CAD build for the part. Positions are in the model's coordinates, mm. A direction names the side the tool comes from. Round coordinates to 2 decimals unless told otherwise and drop trailing zeros. Loops run counter-clockwise (first coordinate to the right, second up) from the corner with the lowest first, then second, coordinate; pieces in that order, holes last.
from build123d import *

# Parameters (mm, degrees)
SKETCH2_W           = 6.35
SKETCH2_H           = 152.4
SKETCH2_H_2         = 6.35
SKETCH2_W_2         = 25.4
SKETCH2_W_3         = 3.175
BOSS_EXTRUDE1_DEPTH = 152.4
SKETCH3_W           = 228.6
SKETCH3_H           = 165.1
BOSS_EXTRUDE2_DEPTH = 12.7


with BuildPart() as part:
    # Sketch2 → Boss-Extrude1 (new body)
    with BuildSketch(Plane.XY):
        with Locations((-111.125, 79.375)):
            Rectangle(SKETCH2_W, SKETCH2_H)
        with Locations((-111.125, 158.75)):
            Rectangle(SKETCH2_W, SKETCH2_H_2)
        with Locations((-95.25, 158.75)):
            Rectangle(SKETCH2_W_2, SKETCH2_H_2)
        with Locations((-80.9625, 158.75)):
            Rectangle(SKETCH2_W_3, SKETCH2_H_2)
        with Locations((-76.2, 158.75)):
            Rectangle(SKETCH2_W, SKETCH2_H_2)
        with Locations((-71.4375, 158.75)):
            Rectangle(SKETCH2_W_3, SKETCH2_H_2)
        with Locations((-57.15, 158.75)):
            Rectangle(SKETCH2_W_2, SKETCH2_H_2)
        with Locations((-42.8625, 158.75)):
            Rectangle(SKETCH2_W_3, SKETCH2_H_2)
        with Locations((-42.8625, 152.4)):
            Rectangle(SKETCH2_W_3, SKETCH2_H_2)
        with Locations((-38.1, 158.75)):
            Rectangle(SKETCH2_W, SKETCH2_H_2)
        with Locations((-33.3375, 158.75)):
            Rectangle(SKETCH2_W_3, SKETCH2_H_2)
        with Locations((-33.3375, 152.4)):
            Rectangle(SKETCH2_W_3, SKETCH2_H_2)
        with Locations((-19.05, 158.75)):
            Rectangle(SKETCH2_W_2, SKETCH2_H_2)
        with Locations((-4.7625, 158.75)):
            Rectangle(SKETCH2_W_3, SKETCH2_H_2)
        with Locations((-4.7625, 152.4)):
            Rectangle(SKETCH2_W_3, SKETCH2_H_2)
        with Locations((0, 158.75)):
            Rectangle(SKETCH2_W, SKETCH2_H_2)
        with Locations((4.7625, 158.75)):
            Rectangle(SKETCH2_W_3, SKETCH2_H_2)
        with Locations((4.7625, 152.4)):
            Rectangle(SKETCH2_W_3, SKETCH2_H_2)
        with Locations((19.05, 158.75)):
            Rectangle(SKETCH2_W_2, SKETCH2_H_2)
        with Locations((33.3375, 158.75)):
            Rectangle(SKETCH2_W_3, SKETCH2_H_2)
        with Locations((38.1, 158.75)):
            Rectangle(SKETCH2_W, SKETCH2_H_2)
        with Locations((33.3375, 152.4)):
            Rectangle(SKETCH2_W_3, SKETCH2_H_2)
        with Locations((42.8625, 152.4)):
            Rectangle(SKETCH2_W_3, SKETCH2_H_2)
        with Locations((42.8625, 158.75)):
            Rectangle(SKETCH2_W_3, SKETCH2_H_2)
        with Locations((57.15, 158.75)):
            Rectangle(SKETCH2_W_2, SKETCH2_H_2)
        with Locations((71.4375, 158.75)):
            Rectangle(SKETCH2_W_3, SKETCH2_H_2)
        with Locations((71.4375, 152.4)):
            Rectangle(SKETCH2_W_3, SKETCH2_H_2)
        with Locations((76.2, 158.75)):
            Rectangle(SKETCH2_W, SKETCH2_H_2)
        with Locations((80.9625, 158.75)):
            Rectangle(SKETCH2_W_3, SKETCH2_H_2)
        with Locations((80.9625, 152.4)):
            Rectangle(SKETCH2_W_3, SKETCH2_H_2)
        with Locations((95.25, 158.75)):
            Rectangle(SKETCH2_W_2, SKETCH2_H_2)
        with Locations((111.125, 158.75)):
            Rectangle(SKETCH2_W, SKETCH2_H_2)
        with Locations((111.125, 79.375)):
            Rectangle(SKETCH2_W, SKETCH2_H)
        with Locations((-111.125, 0)):
            Rectangle(SKETCH2_W, SKETCH2_H_2)
        with Locations((-95.25, 0)):
            Rectangle(SKETCH2_W_2, SKETCH2_H_2)
        with Locations((-80.9625, 0)):
            Rectangle(SKETCH2_W_3, SKETCH2_H_2)
        with Locations((-80.9625, 6.35)):
            Rectangle(SKETCH2_W_3, SKETCH2_H_2)
        with Locations((-76.2, 0)):
            Rectangle(SKETCH2_W, SKETCH2_H_2)
        with Locations((-71.4375, 0)):
            Rectangle(SKETCH2_W_3, SKETCH2_H_2)
        with Locations((-71.4375, 6.35)):
            Rectangle(SKETCH2_W_3, SKETCH2_H_2)
        with Locations((-57.15, 0)):
            Rectangle(SKETCH2_W_2, SKETCH2_H_2)
        with Locations((-42.8625, 0)):
            Rectangle(SKETCH2_W_3, SKETCH2_H_2)
        with Locations((-42.8625, 6.35)):
            Rectangle(SKETCH2_W_3, SKETCH2_H_2)
        with Locations((-38.1, 0)):
            Rectangle(SKETCH2_W, SKETCH2_H_2)
        with Locations((-33.3375, 0)):
            Rectangle(SKETCH2_W_3, SKETCH2_H_2)
        with Locations((-33.3375, 6.35)):
            Rectangle(SKETCH2_W_3, SKETCH2_H_2)
        with Locations((-19.05, 0)):
            Rectangle(SKETCH2_W_2, SKETCH2_H_2)
        with Locations((-4.7625, 0)):
            Rectangle(SKETCH2_W_3, SKETCH2_H_2)
        with Locations((-4.7625, 6.35)):
            Rectangle(SKETCH2_W_3, SKETCH2_H_2)
        Rectangle(SKETCH2_W, SKETCH2_H_2)
        with Locations((4.7625, 0)):
            Rectangle(SKETCH2_W_3, SKETCH2_H_2)
        with Locations((4.7625, 6.35)):
            Rectangle(SKETCH2_W_3, SKETCH2_H_2)
        with Locations((19.05, 0)):
            Rectangle(SKETCH2_W_2, SKETCH2_H_2)
        with Locations((111.125, 0)):
            Rectangle(SKETCH2_W, SKETCH2_H_2)
        with Locations((95.25, 0)):
            Rectangle(SKETCH2_W_2, SKETCH2_H_2)
        with Locations((80.9625, 0)):
            Rectangle(SKETCH2_W_3, SKETCH2_H_2)
        with Locations((80.9625, 6.35)):
            Rectangle(SKETCH2_W_3, SKETCH2_H_2)
        with Locations((71.4375, 6.35)):
            Rectangle(SKETCH2_W_3, SKETCH2_H_2)
        with Locations((76.2, 0)):
            Rectangle(SKETCH2_W, SKETCH2_H_2)
        with Locations((71.4375, 0)):
            Rectangle(SKETCH2_W_3, SKETCH2_H_2)
        with Locations((57.15, 0)):
            Rectangle(SKETCH2_W_2, SKETCH2_H_2)
        with Locations((42.8625, 6.35)):
            Rectangle(SKETCH2_W_3, SKETCH2_H_2)
        with Locations((33.3375, 6.35)):
            Rectangle(SKETCH2_W_3, SKETCH2_H_2)
        with Locations((33.3375, 0)):
            Rectangle(SKETCH2_W_3, SKETCH2_H_2)
        with Locations((38.1, 0)):
            Rectangle(SKETCH2_W, SKETCH2_H_2)
        with Locations((42.8625, 0)):
            Rectangle(SKETCH2_W_3, SKETCH2_H_2)
        with Locations((-80.9625, 152.4)):
            Rectangle(SKETCH2_W_3, SKETCH2_H_2)
        with Locations((-71.4375, 152.4)):
            Rectangle(SKETCH2_W_3, SKETCH2_H_2)
    extrude(amount=BOSS_EXTRUDE1_DEPTH)

    # Sketch3 → Boss-Extrude2 (add)
    with BuildSketch(Plane(origin=(0, 0, 0), x_dir=(-1, 0, 0), z_dir=(0, 0, -1))):
        with Locations((0, 79.375)):
            Rectangle(SKETCH3_W, SKETCH3_H)
    extrude(amount=BOSS_EXTRUDE2_DEPTH)


solid = part.part
Item 1: Flat gauge pin, fed straight in: P1, Ø12, axis at x = 79.5, y = 48, coming from the +Z side. Where does the tip first touch, or does it go through?
Verdict:
P1: stops at z = 0
Item 2: Cut at A-A (y = 30). List the corners of the cut face in (x, z).
Verdict:
outline: (-114.3, -12.7) - (114.3, -12.7) - (114.3, 152.4) - (107.95, 152.4) - (107.95, 0) - (-107.95, 0) - (-107.95, 152.4) - (-114.3, 152.4) - close
Item 3: Wall check: L1, parallel to X at y = 129.5, z = 59; L2, parallel to Y at x = -23, z = 82 (3 decimals); L3, parallel to Z at x = 1.5, y = 7. Give the ranges that are in metal, low to high.
Verdict:
L1: x = -114.3 to -107.95, 107.95 to 114.3
L2: y = -3.175 to 3.175, 155.575 to 161.925
L3: z = -12.7 to 0
Item 4: 3-axis set-ups, long thin cutter, end or side, ignore diameter. For faces 5 (the flat face through (19, 155.575, 75)), 6 (the flat face through (2, 161.925, 71)): which of +Z, -Z, +X, -X, +Y, -Y reach the whole face in a straight line?
Verdict:
face 5: +Z
face 6: +Z, -Z, +X, -X, +Y
Item 5: Mould opens along X. For faces 1 (the flat face through (-9, 0, 152.4)), 2 (the flat face through (114.3, 78, 71)), 3 (the flat face through (19, 3.175, 75)), 4 (the flat face through (-114.3, 78, 71)) say: released by +X, released by -X, zero draft, split by the parting line, or undercut.
Verdict:
face 1: zero draft
face 2: released by +X
face 3: undercut
face 4: released by -X
Item 6: Cut at B-B (x = -50). List the corners of the cut face in (y, z) (3 decimals), plus the area to 3 significant figures.
Verdict:
outline: (-3.175, -12.7) - (161.925, -12.7) - (161.925, 152.4) - (155.575, 152.4) - (155.575, 0) - (3.175, 0) - (3.175, 152.4) - (-3.175, 152.4) - close
area: 4,030 mm2
